The model under review builds one solid part; all positions refer to its coordinate system, in mm. Face numbers are marked on the shaded views. Coordinates: 2 decimals unless noted, no trailing zeros. Loops run counter-clockwise (first coordinate to the right, second up) from the corner with the lowest first, then second, coordinate; pieces in that order, holes last. Notation, with made-up numbers: (-23, 58.5) - (10, 58.5) arc R18 ccw to (10, 92.5) - close; hole circle Ø2 at (23, 53). An arc over 180 degrees is marked (long way). Answer in a Markdown table with one row per item. Add a question column.
(1) Mouldability with a two-part tool opening along Y and no side actions: class the marked faces 1, 2 and 3 as +Y half, -Y half, draft (parallel to the pull), parting line (faces both ways), or undercut.
(2) We need section C-C on z = 13. Write out the cut boundary in (x, y), plus the area to 3 significant figures.
(3) For line 1 along X through (y, z) = (61, -0.5); line 2 along Y through (x, z) = (23.5, 17), list the stretches that pass through material, from the lowest coordinate up.
(4) We need section B-B on z = 0. Write out the cut boundary in (x, y), plus the area to 3 significant figures.
(5) For P1, Ø2, axis at x = 42, z = 9, coming from the +Y side; P2, Ø20, axis at x = 18.5, z = 3, coming from the -Y side, all flat-tipped, find the tip position at first contact; note any pin that passes through.
(6) We need section A-A on x = 85. Write out the cut boundary in (y, z), plus the area to 3 significant figures.
from build123d import *

# Parameters (mm, degrees)
SKETCH_1_W      = 220
SKETCH_1_H      = 120
EXTRUDE_1_DEPTH = 20
EXTRUDE_START   = 60
SKETCH_2_R      = 5
EXTRUDE_2_DEPTH = 8
EXTRUDE_START_2 = -68
SKETCH_3_R      = 5
EXTRUDE_3_DEPTH = 8


with BuildPart() as part:
    # ｽｹｯﾁ1 → ﾎﾞｽ - 押し出し1 (new, symmetric)
    with BuildSketch(Plane.XY):
        Rectangle(SKETCH_1_W, SKETCH_1_H)
    extrude(amount=EXTRUDE_1_DEPTH, both=True)

    # ｽｹｯﾁ2 → ﾎﾞｽ - 押し出し2 (add)
    with BuildSketch(Plane(origin=(0, 0, 0), x_dir=(1, 0, 0), z_dir=(0, 1, 0)).offset(EXTRUDE_START)):
        with Locations(Location((85, 0, 0), (0, 0, 90))):
            Circle(SKETCH_2_R)
        with Locations(Location((-85, 0, 0), (0, 0, 90))):
            Circle(SKETCH_2_R)
    extrude(amount=EXTRUDE_2_DEPTH)

    # ｽｹｯﾁ3 → ﾎﾞｽ - 押し出し3 (add)
    with BuildSketch(Plane(origin=(0, 0, 0), x_dir=(1, 0, 0), z_dir=(0, 1, 0)).offset(EXTRUDE_START_2)):
        with Locations(Location((85, 0, 0), (0, 0, 90))):
            Circle(SKETCH_3_R)
        with Locations(Location((-85, 0, 0), (0, 0, 90))):
            Circle(SKETCH_3_R)
    extrude(amount=EXTRUDE_3_DEPTH)


solid = part.part
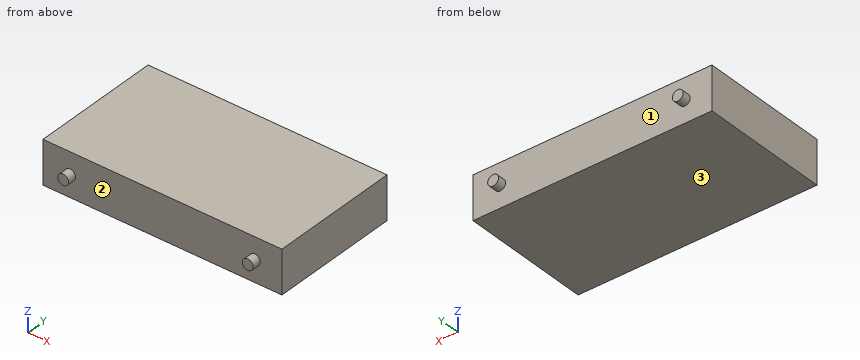
Outcome:
| question | item | result |
|---|---|---|
| 1 | face 1 | +Y half |
| 1 | face 2 | -Y half |
| 1 | face 3 | draft |
| 2 | outline | (-110, -60) - (110, -60) - (110, 60) - (-110, 60) - close |
| 2 | area | 26,400 mm² |
| 3 | line 1 | -89.97 to -80.03, 80.03 to 89.97 |
| 3 | line 2 | -60 to 60 |
| 4 | outline | (-110, -60) - (-90, -60) - (-90, -68) - (-80, -68) - (-80, -60) - (80, -60) - (80, -68) - (90, -68) - (90, -60) - (110, -60) - (110, 60) - (90, 60) - (90, 68) - (80, 68) - (80, 60) - (-80, 60) - (-80, 68) - (-90, 68) - (-90, 60) - (-110, 60) - close |
| 4 | area | 26,700 mm² |
| 5 | P1 | y = 60 |
| 5 | P2 | y = -60 |
| 6 | outline | (-68, -5) - (-60, -5) - (-60, -20) - (60, -20) - (60, -5) - (68, -5) - (68, 5) - (60, 5) - (60, 20) - (-60, 20) - (-60, 5) - (-68, 5) - close |
| 6 | area | 4,960 mm² |
